Autodesk Inventor part; units mm, degrees
ref_plane "XZ Plane" through (0, 0, 0) normal (0, 1, 0) x (-1, 0, 0)
ref_plane "XY Plane" through (0, 0, 0) normal (0, 0, 1) x (1, 0, 0)
sketch "Sketch1" plane through (0, 0, 0) normal (0, 1, 0) x (-1, 0, 0)
  line L0 (-273.05, 301.625) -> (-273.05, -301.625)
  line L1 (-273.05, -301.625) -> (273.05, -301.625)
  line L2 (273.05, -301.625) -> (273.05, 301.625)
  line L3 (273.05, 301.625) -> (-273.05, 301.625)
  line L4 (-273.05, 301.625) -> (273.05, -301.625) construction
  line L5 (-273.05, -301.625) -> (273.05, 301.625) construction
  point P0 (0, 0)
  dimension "baseLength" = 603.25
  dimension "baseWidth" = 546.1
extrude "Extrusion1" add sketch "Sketch1" along normal blind 17.78
sketch "Sketch2" plane through (0, 0, 0) normal (0, -1, 0) x (1, 0, 0)
  line L0 (273.05, 301.625) -> (273.05, -301.625)
  line L1 (273.05, 193.675) -> (222.25, 193.675)
  line L2 (222.25, 193.675) -> (222.25, 92.075)
  line L3 (222.25, 92.075) -> (273.05, 92.075)
  line L4 (273.05, 92.075) -> (273.05, 193.675)
  line L5 (-273.05, 301.625) -> (273.05, 301.625)
  point P0 (0, 0)
  dimension "backToEndOfGearBox" = 107.95
  dimension "backToFrontOfGearBox" = 209.55
  dimension "wdithForGearBox" = 50.8
extrude "Extrusion2" cut sketch "Sketch2" against normal through all
mirror "Mirror1" about plane through (0, 0, 0) normal (1, 0, 0) of "Extrusion2"
sketch "Sketch3" plane through (0, 17.78, 0) normal (0, 1, 0) x (1, 0, 0)
  line L0 (273.05, -263.525) -> (260.35, -263.525)
  line L1 (260.35, -263.525) -> (260.35, -238.125)
  line L2 (260.35, -238.125) -> (273.05, -238.125)
  line L3 (273.05, -238.125) -> (273.05, -263.525)
  line L4 (273.05, -301.625) -> (273.05, -193.675)
  line L5 (-273.05, -301.625) -> (273.05, -301.625)
  point P0 (0, 0)
  dimension "d9" = 25.4
  dimension "d10" = 12.7
  dimension "d11" = 38.1
extrude "Extrusion3" cut sketch "Sketch3" against normal through all
mirror "Mirror2" about plane through (0, 0, 0) normal (1, 0, 0) of "Extrusion3"
sketch "Sketch4" plane through (0, 17.78, 0) normal (0, 1, 0) x (1, 0, 0)
  line L0 (273.05, -92.075) -> (273.05, 301.625)
  line L1 (273.05, -34.925) -> (260.35, -34.925)
  line L2 (260.35, -34.925) -> (260.35, -9.525)
  line L3 (260.35, -9.525) -> (273.05, -9.525)
  line L4 (273.05, -9.525) -> (273.05, -34.925)
  line L5 (-273.05, -301.625) -> (273.05, -301.625)
  point P0 (0, 0)
  dimension "d14" = 25.4
  dimension "d15" = 266.7
  dimension "d16" = 12.7
extrude "Extrusion4" cut sketch "Sketch4" against normal through all
mirror "Mirror3" about plane through (0, 0, 0) normal (1, 0, 0) of "Extrusion4"
sketch "Sketch5" plane through (0, 17.78, 0) normal (0, 1, 0) x (1, 0, 0)
  line L0 (273.05, 269.875) -> (260.35, 269.875)
  line L1 (260.35, 269.875) -> (260.35, 301.625)
  line L2 (260.35, 301.625) -> (273.05, 301.625)
  line L3 (273.05, 301.625) -> (273.05, 269.875)
  line L4 (273.05, -9.525) -> (273.05, 301.625)
  line L5 (273.05, 301.625) -> (-273.05, 301.625)
  point P0 (0, 0)
  dimension "d19" = 12.7
  dimension "d20" = 31.75
extrude "Extrusion5" cut sketch "Sketch5" against normal through all
mirror "Mirror4" about plane through (0, 0, 0) normal (1, 0, 0) of "Extrusion5"
sketch "Sketch8" plane through (0, 17.78, 0) normal (0, 1, 0) x (1, 0, 0)
  line L0 (-76.2, 301.625) -> (76.2, 301.625)
  line L1 (76.2, 301.625) -> (76.2, 136.525)
  line L2 (76.2, 136.525) -> (-76.2, 136.525)
  line L3 (-76.2, 136.525) -> (-76.2, 301.625)
  line L4 (260.35, 301.625) -> (-260.35, 301.625)
  point P0 (0, 0)
  dimension "d23" = 76.2
  dimension "d24" = 76.2
  dimension "d25" = 165.1
extrude "Extrusion6" cut sketch "Sketch8" against normal through all
equation "\"baseLength\" = userBaseLength"
equation "\"baseWidth\" = userBaseWidth"
equation "\"d9\" = lengthOfSpacingForBolt"
equation "\"d10\" = widthOfSpacingForBolt"
equation "\"d11\" = distanceFromBackForEndBolt"
equation "\"d14\" = lengthOfSpacingForBolt"
equation "\"d16\" = widthOfSpacingForBolt"
equation "\"d19\" = widthOfSpacingForBolt"
equation "\"spaceingAlongSides\" = 3.175"
equation "\"distanceFromBackForEndBolt\" = 38.1"
equation "\"widthOfSpacingForBolt\" = 12.7"
equation "\"lengthOfSpacingForBolt\" = 25.4"
equation "\"userBaseLength\" = 603.25"
equation "\"userBaseWidth\" = 546.1"
properties part number "RhinoBottomFloorPlate01-ExtendedBy3Inches" material "Wood (Birch)"
Work out the finished part from the listing and answer in its coordinate system (mm). A direction names the side the tool comes from. Give positions to 0.01 mm unless a question says otherwise; leave off trailing zeros. Order: outer loops, then holes, each group sorted by start corner. A loop starts at its lowest first (then second) coordinate and runs counter-clockwise, first axis right, second up. Notation, with made-up numbers: (-40, 82) - (-32, 82) arc R32 cw to (-32, 116) - close; hole circle Ø5 at (20.25, 26). An arc over 180 degrees is marked (long way). One line per item, written item: value. Start each with the question number.
1. Each of these flat-tipped pins is pushed along its axis until it touches: pin 1 Ø10 at (x, y) = (-268, 7) entering from -Z (3 decimals); pin 2 Ø9 at (x, y) = (27, 12) entering from -Z (3 decimals); pin 3 Ø5.5 at (y, z) = (6, 249) entering from +X; pin 4 Ø5 at (y, z) = (15, 94.5) entering from +X. Where does it stop, or does it pass through?
2. For a pull along Z with two mould halves and no side action, classify faces 1 (the face through (222.25, 9, 144)), 2 (the face through (-4, 9, 301.625)), 3 (the face through (-273.05, 9, 216)), 4 (the face through (267, 9, 34.925)) as released by +Z, released by -Z, zero draft, split by the parting line, or undercut.
3. Consider line 1 (X direction, y = 9.5, z = -236.5); line 2 (Z direction, x = 22, y = 15.25) (3 decimals); line 3 (X direction, y = 11, z = 12.5). Determine where each line is inside the solid, lowest interval first.
4. Which of the six approach directions +Z, -Z, +X, -X, +Y, -Y give full straight-line access (tool end or side, diameter ignored) to faces 5 (the face through (248, 9, 193.675)), 6 (the face through (-222.25, 9, 142)), 7 (the face through (260.35, 9, -286))?
5. Section A-A, the plane z = -163 is taken. Write down the section's boundary in (x, y).
6. Section B-B, the plane x = 65.5 is taken. Write down the section's boundary in (y, z) (3 decimals).
7. Section C-C, the plane z = 246.5 is taken. Write down the section's boundary in (x, y), then the cut area to 3 significant figures.
Filled sheet:
1. pin 1: z = -269.875
1. pin 2: z = -136.525
1. pin 3: x = 260.35
1. pin 4: x = 273.05
2. face 1: undercut
2. face 2: released by +Z
2. face 3: zero draft
2. face 4: undercut
3. line 1: -273.05 to -76.2, 76.2 to 273.05
3. line 2: -136.525 to 301.625
3. line 3: -260.35 to 260.35
4. face 5: +X, +Y, -Y
4. face 6: -X, +Y, -Y
4. face 7: -Z, +X, +Y, -Y
5. outline: (-273.05, 0) - (-76.2, 0) - (-76.2, 17.78) - (-273.05, 17.78) - close; (76.2, 0) - (273.05, 0) - (273.05, 17.78) - (76.2, 17.78) - close
6. outline: (0, -136.525) - (17.78, -136.525) - (17.78, 301.625) - (0, 301.625) - close
7. outline: (-260.35, 0) - (260.35, 0) - (260.35, 17.78) - (-260.35, 17.78) - close
7. area: 9,260 mm²
